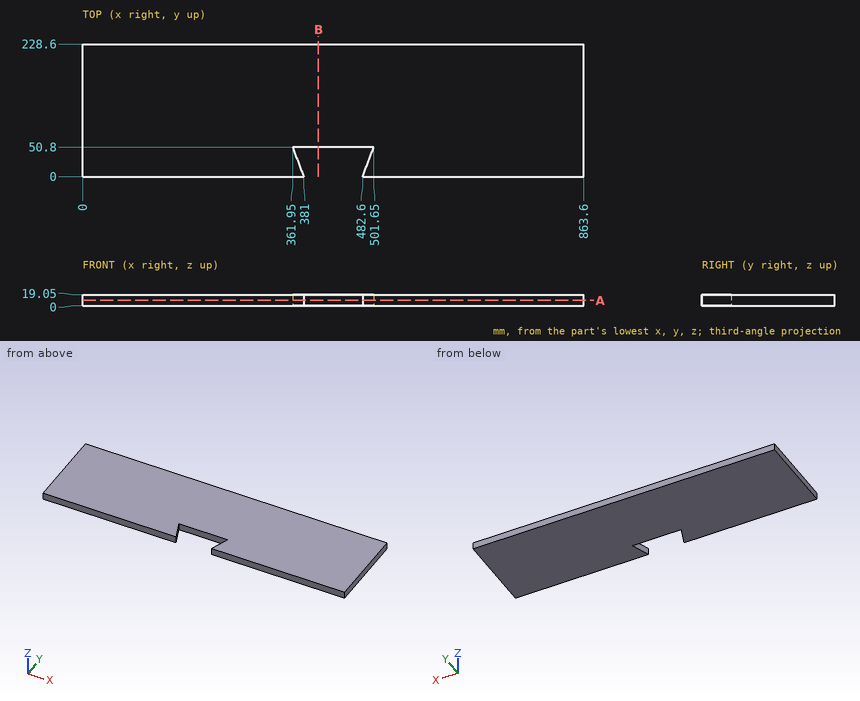
Design review of the part shown in the three views and the two pictorial views. Dimensions are in mm from the part's minimum x, y and z. Round coordinates to 2 decimals unless told otherwise and drop trailing zeros. Write each loop counter-clockwise with the first axis right and the second up, starting at its lowest first coordinate (ties: lowest second). Pieces come first, ordered by that corner, then holes.
1) Take a section at B-B on x = 406.5. Give the boundary of the cut face in (y, z).
Answer below:
outline: (50.8, 0) - (228.6, 0) - (228.6, 19.05) - (50.8, 19.05) - close
2) Take a section at A-A on z = 9.25. Give the boundary of the cut face in (x, y).
Answer below:
outline: (0, 0) - (381, 0) - (361.95, 50.8) - (501.65, 50.8) - (482.6, 0) - (863.6, 0) - (863.6, 228.6) - (0, 228.6) - close
3) For line 1 along Y through (x, z) = (437.5, 11.5); line 2 along X through (y, z) = (27, 15.75) (3 decimals), list the stretches that pass through material, from the lowest coordinate up.
Answer below:
line 1: y = 50.8 to 228.6
line 2: x = 0 to 370.875, 492.725 to 863.6
4) Insertion check: pin 1 Ø10 at (x, z) = (418, 8) entering from -Y. The pin has a flat end and moves straight along its axis. Give the tip position at first contact, or say it passes through.
Answer below:
pin 1: stops at y = 50.8
